```python
from build123d import *

# Parameters (mm, degrees)
SKETCH_1_W          = 2252
SKETCH_1_H          = 100
EXTRUDE_1_DEPTH     = 8
SKETCH_2_W          = 2252
SKETCH_2_H          = 8
EXTRUDE_2_DEPTH     = 92
CUT_EXTRUDE_3_DEPTH = 1135.846245092


with BuildPart() as part:
    # 草图1 → 凸台-拉伸1 (new body)
    with BuildSketch(Plane.XY):
        with Locations((0, 50)):
            Rectangle(SKETCH_1_W, SKETCH_1_H)
    extrude(amount=EXTRUDE_1_DEPTH)

    # 草图2 → 凸台-拉伸2 (add)
    with BuildSketch(Plane.XY.offset(8)):
        with Locations((0, 96)):
            Rectangle(SKETCH_2_W, SKETCH_2_H)
    extrude(amount=EXTRUDE_2_DEPTH)

    # 草图3 → 切除-拉伸3 (cut, through all)
    with BuildSketch(Plane(origin=(0, 100, 0), x_dir=(1, 0, 0), z_dir=(0, 1, 0))):
        Polygon((886, -100), (1126, 0), (1126, -100), align=None)
    cut_extrude_3 = extrude(amount=-CUT_EXTRUDE_3_DEPTH, mode=Mode.SUBTRACT)

    # 镜向8: 切除-拉伸3 across plane
    add(cut_extrude_3.mirror(Plane(origin=(0, 0, 0), x_dir=(0, 0, 1), z_dir=(1, 0, 0))), mode=Mode.SUBTRACT)


solid = part.part
```
Input: part model. Units: mm. Frame: model coordinates. A direction names the side the tool comes from. Coordinates: 2 decimals unless noted, no trailing zeros. Order: outer loops, then holes, each group sorted by start corner. A loop starts at its lowest first (then second) coordinate and runs counter-clockwise, first axis right, second up. Notation, with made-up numbers: (0.5, 44) - (27.5, 44) arc R10 ccw to (27.5, 54) - close; hole circle Ø10 at (70.25, 28.5). An arc over 180 degrees is marked (long way). Put each result on its own line as item: value.
1. Cut plane C-C on y = 35.5. Return the cut outline in (x, z), then the cut area to 3 significant figures.
Report:
outline: (-1126, 0) - (1126, 0) - (1106.8, 8) - (-1106.8, 8) - close
area: 17,900 mm2
2. Draft query along Z for faces 3 (the face through (-16, 100, 49)), 4 (the face through (-1058.8, 94.7, 28)), 5 (the face through (-16, 51, 0)). Return one class per face: pulls with the +Z half, pulls with the -Z half, needs draft (parallel to the pull), parting line crosses it, or undercut.
Report:
face 3: needs draft
face 4: pulls with the +Z half
face 5: pulls with the -Z half
3. Cut plane B-B on z = 36. Return the cut outline in (x, y).
Report:
outline: (-1039.6, 92) - (1039.6, 92) - (1039.6, 100) - (-1039.6, 100) - close
4. Cut plane D-D on x = 968.5. Return the cut outline in (y, z) (3 decimals).
Report:
outline: (0, 0) - (100, 0) - (100, 65.625) - (92, 65.625) - (92, 8) - (0, 8) - close
5. Cut plane A-A on x = -422.5. Return the cut outline in (y, z).
Report:
outline: (0, 0) - (100, 0) - (100, 100) - (92, 100) - (92, 8) - (0, 8) - close
6. Contact query for flat-ended pins moving along their axis: pin 1 Ø10 at (y, z) = (12, 13.5) entering from -X; pin 2 Ø8 at (x, y) = (-818, 81) entering from +Z; pin 3 Ø2 at (x, z) = (-230.5, 85.5) entering from -Y. Output: stop coordinate, or through.
Report:
pin 1: passes through
pin 2: stops at z = 8
pin 3: stops at y = 92
7. Line query: line 1 along Z through (x, y) = (-1015, 59.5); line 2 along Y through (x, z) = (732.5, 84.5). Output: solid intervals per line, ascending.
Report:
line 1: z = 0 to 8
line 2: y = 92 to 100
8. Reachability of faces 1 (the face through (1058.8, 94.7, 28)), 2 (the face through (-15, 47, 8)) from +Z, -Z, +X, -X, +Y, -Y: full face, straight path, thin tool, end or side. Return the list, or none.
Report:
face 1: +Z, +X, +Y, -Y
face 2: +Z, +X, -X, -Y
